```python
from build123d import *

# Parameters (mm, degrees)
SKETCH_2_R               = 1.6
CUT_EXTRUDE_1_DEPTH      = 3
PATTERN_CIRCULAR_1_COUNT = 4
CHAMFER_1_SIZE           = 0.4


with BuildPart() as part:
    # Эскиз1 → Повернуть1 (revolve)
    with BuildSketch(Plane(origin=(0, 0, 0), x_dir=(1, 0, 0), z_dir=(0, 1, 0))):
        Polygon((-4, 0), (-18, 0), (-18, 3), (-9.5, 3), (-9.5, 6), (-6, 6), (-6, 1), (-4, 1), align=None)
    revolve(axis=Axis((0, 0, 0), (0, 0, -1)))

    # Эскиз2 → Вырез-Вытянуть1 (cut)
    with BuildSketch(Plane.XY):
        with Locations((10.606601718, 10.606601718)):
            Circle(SKETCH_2_R)
    cut_extrude_1 = extrude(amount=-CUT_EXTRUDE_1_DEPTH, mode=Mode.SUBTRACT)

    # Круговой массив1: Вырез-Вытянуть1 ×4 about axis
    pattern_circular_1_axis = Axis((0, 0, 0), (0, 0, 1))
    for i in range(1, PATTERN_CIRCULAR_1_COUNT):
        add(cut_extrude_1.rotate(pattern_circular_1_axis, i * 360 / PATTERN_CIRCULAR_1_COUNT), mode=Mode.SUBTRACT)

    # Фаска1
    chamfer_1_edges = [part.edges().sort_by_distance(p)[0] for p in [
        (6, 0, -6),
        (9.5, 0, -6),
    ]]
    chamfer(chamfer_1_edges, length=CHAMFER_1_SIZE)


solid = part.part
```
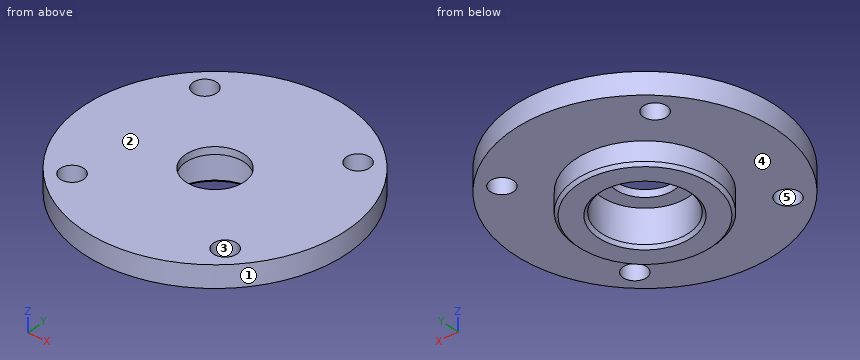
Can you work these out from the model? Positions are in its coordinate system, mm. Face numbers are marked on the shaded views. A direction names the side the tool comes from. Give positions to 0.01 mm unless a question says otherwise; leave off trailing zeros. Loops run counter-clockwise (first coordinate to the right, second up) from the corner with the lowest first, then second, coordinate; pieces in that order, holes last. Notation, with made-up numbers: M 66,83 L 119,83 A28 ccw 119,101 Z; hole C -13,-11.75 d3. An arc over 180 degrees is marked long. Answer in a Markdown table with one row per item.
1. Thinking about a two-plate mould opening in X: for the marked faces 1, 2 and 3, which applies, released by +X, released by -X, zero draft, split by the parting line, or undercut?
Taken from the geometry:
| item | result |
|---|---|
| face 1 | split by the parting line |
| face 2 | zero draft |
| face 3 | undercut |
2. If I drill on line 1 along Y through (x, z) = (-9.5, -1.25); line 2 along Y through (x, z) = (-10.5, -1.7); line 3 along Z through (x, y) = (-5, -15), over which ranges is the centre line in solid material (lowest first)?
Taken from the geometry:
| item | result |
|---|---|
| line 1 | y = -15.29 to -11.76, -9.45 to 9.45, 11.76 to 15.29 |
| line 2 | y = -14.62 to -12.2, -9.01 to 9.01, 12.2 to 14.62 |
| line 3 | z = -3 to 0 |
3. For pin 1 Ø2 at (y, z) = (-2, -2.5) entering from +X; pin 2 Ø5 at (x, y) = (10.61, 10.61) entering from -Z; pin 3 Ø3 at (y, z) = (4, -4) entering from -X; pin 4 Ø13 at (x, y) = (-0.5, -2) entering from -Z, each with a flat end and sliding along its axis, tell me the tip position at first contact or that it passes through.
Taken from the geometry:
| item | result |
|---|---|
| pin 1 | stops at x = 17.97 |
| pin 2 | stops at z = -3 |
| pin 3 | stops at x = -17.77 |
| pin 4 | stops at z = -6 |
4. Suppose I cut it at C-C on z = -4.05. Write out the boundary of the cut face in (x, y).
Taken from the geometry:
| item | result |
|---|---|
| outline | C 0,0 d19; hole C 0,0 d12 |
5. Suppose I cut it at A-A on x = 0. Write out the boundary of the cut face in (y, z), plus the area to 3 significant figures.
Taken from the geometry:
| item | result |
|---|---|
| outline | M -18,-3 L -9.5,-3 L -9.5,-5.6 L -9.1,-6 L -6.4,-6 L -6,-5.6 L -6,-1 L -4,-1 L -4,0 L -18,0 Z; M 4,-1 L 6,-1 L 6,-5.6 L 6.4,-6 L 9.1,-6 L 9.5,-5.6 L 9.5,-3 L 18,-3 L 18,0 L 4,0 Z |
| area | 96.7 mm² |
6. Which directions (+Z, -Z, +X, -X, +Y, -Y) give clear straight access to the entire face, cutting with the end or side of a thin tool? Please do the marked faces 4 and 5.
Taken from the geometry:
| item | result |
|---|---|
| face 4 | -Z |
| face 5 | +Z, -Z |
7. Suppose I cut it at D-D on y = 13. Write out the boundary of the cut face in (x, z), plus the area to 3 significant figures.
Taken from the geometry:
| item | result |
|---|---|
| outline | M -12.45,-3 L 12.45,-3 L 12.45,0 L -12.45,0 Z |
| area | 74.7 mm² |
